Autodesk Inventor part; units mm, degrees
ref_plane "YZ Plane" through (0, 0, 0) normal (1, 0, 0) x (0, 1, 0)
ref_plane "XZ Plane" through (0, 0, 0) normal (0, 1, 0) x (-1, 0, 0)
ref_plane "XY Plane" through (0, 0, 0) normal (0, 0, 1) x (1, 0, 0)
sketch "スケッチ1" plane through (0, 0, 0) normal (0, 0, 1) x (1, 0, 0)
  line L0 (-16, 21.5) -> (-10.583, 21.5) construction
  line L1 (16, 21.5) -> (16, 9.5) construction
  line L2 (16, -21.5) -> (-16, -21.5)
  line L3 (-16, -21.5) -> (-16, 9.5)
  line L4 (-16, 21.5) -> (16, -21.5) construction
  line L5 (16, 21.5) -> (-16, -21.5) construction
  line L6 (-14.4, -21.5) -> (-14.4, -30)
  line L7 (-14.4, -30) -> (14.4, -30)
  line L8 (0, 21.5) -> (0, -21.5) construction
  line L9 (14.4, -21.5) -> (14.4, -30)
  line L10 (-13.5, 21.5) -> (-13.5, -21.5) construction
  circle A0 centre (0, 9.5) radius 6
  circle A1 centre (0, 9.5) radius 4
  arc A2 (-10.583, 21.5) -> (-16, 9.5) centre (0, 9.5) ccw
  arc A3 (16, 9.5) -> (10.583, 21.5) centre (0, 9.5) ccw
  line L11 (-10.583, 21.5) -> (10.583, 21.5)
  line L12 (-16, 9.5) -> (-16, 21.5) construction
  line L13 (10.583, 21.5) -> (16, 21.5) construction
  line L14 (16, 9.5) -> (16, -21.5)
  circle A4 centre (0, 9.5) radius 3
  circle A5 centre (0, 9.5) radius 4.8
  point P0 (0, 0)
  point P1 (-13.5, 8.5)
  point P2 (-13.5, -18.5)
  point P3 (13.5, 8.5)
  point P4 (13.5, -18.5)
  dimension "d0" = 32
  dimension "d1" = 43
  dimension "d4" = 28.8
  dimension "d5" = 8.5
  dimension "d8" = 27
  dimension "d9" = 8.5
  dimension "d12" = 18.5
  dimension "d13" = 12
  dimension "d14" = 8
  dimension "d15" = 9.5
  dimension "d17" = 16
  dimension "d32" = 13.5
  dimension "d47" = 6
  dimension "d67" = 9.6
extrude "押し出し1" add sketch "スケッチ1" against normal blind 12.2 contours L2 L3 A2 L11 A3 L14 | A0 | A1 | A4 | A5
extrude "押し出し2" add sketch "スケッチ1" against normal blind 12 contours L9 L7 L6 L2
extrude "押し出し3" add sketch "スケッチ1" against normal blind 14 contours A0 | A1 | A4 | A5
extrude "押し出し4" add sketch "スケッチ1" against normal blind 17.7 contours A1 | A4
chamfer "面取り1" distance 1.2 angle 45 1 edges at (-6, 9.5, -14)
sketch "スケッチ2" plane through (0, 9.5, -17.7) normal (0, 0, -1) x (-1, 0, 0)
  circle A0 centre (0, 0) radius 4
  point P0 (0, -9.5)
hole "穴1" at (0, 9.5, -17.7) direction (0, 0, 1) diameter 2.459 depth 6
extrude "押し出し5" add sketch "スケッチ1" along normal blind 27.3 contours L2 L3 A2 L11 A3 L14 | A0 | A1 | A4 | A5
hole "穴2" at (-13.5, 8.5, 0) at (-13.5, -18.5, 0) at (13.5, 8.5, 0) at (13.5, -18.5, 0) direction (0, 0, 1) diameter 2.7 end through all both
extrude "押し出し6" cut sketch "スケッチ1" against normal blind 0.4 contours L9 L7 L6 L2
fillet "フィレット1" radius 2 2 edges at (16, -21.5, 7.55) (-16, -21.5, 7.55)
extrude "押し出し7" add sketch "スケッチ1" along normal blind 28.2 contours A0 | A1 | A4 | A5
extrude "押し出し8" add sketch "スケッチ1" along normal blind 30.75 contours A4
sketch "スケッチ3" plane through (0, 9.5, 30.75) normal (0, 0, 1) x (1, 0, 0)
  circle A0 centre (0, 0) radius 1.2295
  point P0 (0, -9.5)
hole "穴3" at (0, 9.5, 30.75) direction (0, 0, -1) diameter 2.459 end through all
sketch "スケッチ4" plane through (0, 9.5, 28.2) normal (0, 0, 1) x (1, 0, 0)
  circle A0 centre (0, 0) radius 4
  circle A1 centre (0, 0) radius 3
  point P0 (0, -9.5)
extrude "押し出し9" cut sketch "スケッチ4" against normal blind 2.3
chamfer "面取り2" distance 0.5 angle 45 1 edges at (-3, 9.5, 30.75)
extrude "押し出し10" add sketch "スケッチ1" against normal blind 14.2 contours A5
chamfer "面取り4" distance 0.1 angle 45 2 edges at (-6, 9.5, 28.2) (-4, 9.5, 28.2)
properties part number "B3M-SC-1170-A"
CAD build for the part. Positions are in the model's coordinates, mm. A direction names the side the tool comes from. Round coordinates to 2 decimals unless told otherwise and drop trailing zeros. Write each loop counter-clockwise with the first axis right and the second up, starting at its lowest first coordinate (ties: lowest second). Pieces come first, ordered by that corner, then holes. Notation, with made-up numbers: M -32.5,-39 L -12.5,-39 A17 ccw -12.5,-9 Z; hole C -31.75,10.5 d1. An arc over 180 degrees is marked long. One line per question, with ' | ' between items.
1. Mould opens along X. For faces 4 (the cylindrical face through (-14.638, -17.774, 7.826)), 5 (the cylindrical face through (-14.638, 9.226, 7.826)), 6 (the flat face through (0, 0, -12.2)), 7 (the cylindrical face through (-15.43, -20.9, 7.83)) say: pulls with the +X half, pulls with the -X half, needs draft (parallel to the pull), parting line crosses it, or undercut.
Working result:
face 4: undercut | face 5: undercut | face 6: needs draft | face 7: pulls with the -X half
2. Pin check, flat tips, straight feed: pin 1 Ø12 at (x, z) = (-11.5, 19) entering from -Y; pin 2 Ø4 at (x, y) = (9, -20) entering from +Z; pin 3 Ø1.6 at (x, y) = (13.5, -18.5) entering from -Z; pin 4 Ø6 at (x, y) = (9, -23.5) entering from -Z. Stop position of each tip, or through.
Working result:
pin 1: y = -21.5 | pin 2: z = 27.3 | pin 3: through | pin 4: z = -12.2
3. Cut at A-A on z = 16. Write the cut outline in (x, y).
Working result:
outline: M -16,-19.5 A2 ccw -14,-21.5 L 14,-21.5 A2 ccw 16,-19.5 L 16,9.5 A16 ccw 10.58,21.5 L -10.58,21.5 A16 ccw -16,9.5 Z; hole C -13.5,-18.5 d2.7; hole C -13.5,8.5 d2.7; hole C 0,9.5 d2.46; hole C 13.5,-18.5 d2.7; hole C 13.5,8.5 d2.7
4. Cut at D-D on z = -3.5. Write the cut outline in (x, y), and give its area (3 significant figures).
Working result:
outline: M -16,-19.5 A2 ccw -14.4,-21.46 L -14.4,-30 L 14.4,-30 L 14.4,-21.46 A2 ccw 16,-19.5 L 16,9.5 A16 ccw 10.58,21.5 L -10.58,21.5 A16 ccw -16,9.5 Z; hole C -13.5,-18.5 d2.7; hole C -13.5,8.5 d2.7; hole C 0,9.5 d2.46; hole C 13.5,-18.5 d2.7; hole C 13.5,8.5 d2.7 | area: 1,550 mm2
5. Cut at C-C on x = -8.5. Write the cut outline in (y, z).
Working result:
outline: M -30,-12 L -21.5,-12 L -21.5,-12.2 L 21.5,-12.2 L 21.5,27.3 L -21.5,27.3 L -21.5,-0.4 L -30,-0.4 Z
6. Cut at B-B on y = -18.5. Write the cut outline in (x, z).
Working result:
outline: M -16,-12.2 L -14.85,-12.2 L -14.85,27.3 L -16,27.3 Z; M -12.15,-12.2 L 12.15,-12.2 L 12.15,27.3 L -12.15,27.3 Z; M 14.85,-12.2 L 16,-12.2 L 16,27.3 L 14.85,27.3 Z
7. Which spindle directions (+Z, -Z, +X, -X, +Y, -Y) get a long thin tool onto all of the face, cutting with end or side? Do faces 1 (the flat face through (0, -26, -0.4)), 2 (the flat face through (14.4, -26, -6)), 3 (the flat face through (0, -26, -12)). Say none if no direction does.
Working result:
face 1: +Z, +X, -X, -Y | face 2: +Z, -Z, +X, -Y | face 3: -Z, +X, -X, -Y
8. Probe L1, parallel to X at y = -18.5, z = 11.5; L2, parallel to Y at x = 13.5, z = 18; L3, parallel to Y at x = 0, z = 26. List the from-to ranges inside material, lowest first. Write a range as from..to.
Working result:
L1: -16..-14.85, -12.15..12.15, 14.85..16 | L2: -21.5..-19.85, -17.15..7.15, 9.85..18.09 | L3: -21.5..5.5, 6.5..8.27, 10.73..12.5, 13.5..21.5
